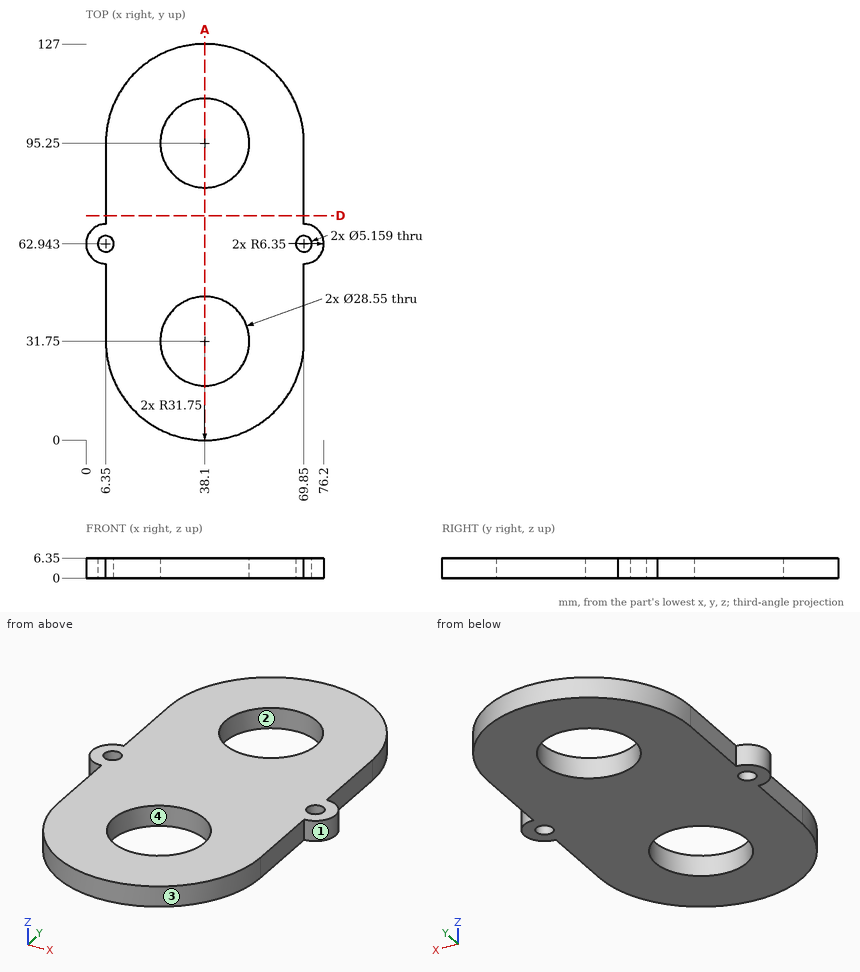
Input: dimensioned drawing with shaded views. Units: mm. Origin: part minimum x, y, z. Give positions to 0.01 mm unless a question says otherwise; leave off trailing zeros. Loops run counter-clockwise (first coordinate to the right, second up) from the corner with the lowest first, then second, coordinate; pieces in that order, holes last. Notation, with made-up numbers: M -28.75,36 L 6.25,36 A17 cw 6.25,54 Z; hole C 57.25,-29.75 d1. An arc over 180 degrees is marked long. Put each result on its own line as item: value. Start each with the question number.
1) Pull-direction query (X, two-part tool) for the marked faces 1, 2, 3 and 4; classes: pulls with the +X half, pulls with the -X half, needs draft (parallel to the pull), parting line crosses it, or undercut.
2) Cut plane A-A (x = 38.1). Give the number of separate pieces and of enclosed holes in the cut face, then the cut area to 3 significant figures.
3) Cut plane D-D (y = 72). Output: boundary loops of the cut face in (x, z).
4) Ray query, line 1 along Y through (x, z) = (38.1, 3.5) (1 decimal); line 2 along Y through (x, z) = (36.5, 1) (1 decimal); line 3 along X through (y, z) = (101, 3.75) (1 decimal). Return the intervals inside material, ascending.
5) Contact query for flat-ended pins moving along their axis: pin 1 (3 mm diameter, centred on x = 26.5, y = 100, fed in from -Z) (1 decimal); pin 2 (3 mm diameter, centred on y = 50, z = 4.5, fed in from -X); pin 3 (1 mm diameter, centred on x = 63.5, z = 3, fed in from -Y); pin 4 (3 mm diameter, centred on y = 38.5, z = 3.5, fed in from +X). Output: stop coordinate, or through.
Verdict:
1. face 1: pulls with the +X half
1. face 2: undercut
1. face 3: parting line crosses it
1. face 4: undercut
2. separate pieces: 3
2. enclosed holes: 0
2. area: 444 mm2
3. outline: M 6.35,0 L 69.85,0 L 69.85,6.35 L 6.35,6.35 Z
4. line 1: 0 to 17.5, 46 to 81, 109.5 to 127
4. line 2: 0 to 17.6, 45.9 to 81.1, 109.4 to 127
4. line 3: 6.9 to 25, 51.2 to 69.3
5. pin 1: through
5. pin 2: x = 6.35
5. pin 3: y = 12.05
5. pin 4: x = 69.85
